Geometry check sheet. Reference: the model listing, model coordinates, mm. A direction names the side the tool comes from. Round coordinates to 2 decimals unless told otherwise and drop trailing zeros. Order: outer loops, then holes, each group sorted by start corner. A loop starts at its lowest first (then second) coordinate and runs counter-clockwise, first axis right, second up. Notation, with made-up numbers: (20.25, 43.5) -> (43.25, 43.5) arc R16 cw to (43.25, 49.5) -> close; hole circle Ø1 at (51, -22.75). An arc over 180 degrees is marked (long way). Answer as a JSON object with one key per item and string values. Group by question number.
from build123d import *

# Parameters (mm, degrees)
EXTRUDE077_DEPTH                     = 23
EXTRUDE077_PLACEMENT_ANGLE           = 45
EXTRUDE076_DEPTH                     = 23
EXTRUDE076_PLACEMENT_ANGLE           = -45
EXTRUDE049_DEPTH                     = 5
SKETCH050_AS_DRAWN_R                 = 10.75
EXTRUDE048_DEPTH                     = 27
EXTRUDE048_ONTO_SKETCH050_ROLL_ANGLE = 90
SKETCH052_R                          = 2.75
EXTRUDE050_DEPTH                     = 3
SKETCH046_R                          = 3.5
SKETCH046_R_2                        = 1.75
SKETCH046_R_3                        = 1.65
EXTRUDE044_DEPTH                     = 30
SKETCH047_AS_DRAWN_R                 = 12.5
EXTRUDE047_DEPTH                     = 50
EXTRUDE047_ONTO_SKETCH047_ROLL_ANGLE = 90
EXTRUDE045_DEPTH                     = 60
SKETCH049_AS_DRAWN_W                 = 50
SKETCH049_AS_DRAWN_H                 = 17.5
EXTRUDE046_DEPTH                     = 78
EXTRUDE046_ONTO_SKETCH049_ROLL_ANGLE = 90
CHAMFER_SIZE                         = 0.5
CHAMFER_PLACEMENT_ANGLE              = 180


with BuildPart() as extrude077:
    # Sketch077 → Extrude077 (new body)
    with BuildSketch(Plane.YZ):
        Polygon((-8.660254, 15), (0, 15), (0, 0), align=None)
    extrude(amount=-EXTRUDE077_DEPTH)


with BuildPart() as extrude077_1:
    # Extrude077 placement: moved
    add(extrude077.part.moved(Location((-13, 0, 0))).rotate(Axis((-13, 0, 0), (0, 0, 1)), EXTRUDE077_PLACEMENT_ANGLE))


with BuildPart() as fusion032:
    # Sketch077 → Extrude076 (new body)
    with BuildSketch(Plane.YZ):
        Polygon((-8.660254, 15), (0, 15), (0, 0), align=None)
    extrude(amount=EXTRUDE076_DEPTH)


with BuildPart() as fusion032_1:
    # Extrude076 placement: moved
    add(fusion032.part.moved(Location((13, 0, 0))).rotate(Axis((13, 0, 0), (0, 0, 1)), EXTRUDE076_PLACEMENT_ANGLE))

    # Fusion032: union Extrude077
    add(extrude077_1.part)


with BuildPart() as fusion032_2:
    # Fusion032 placement: moved
    add(fusion032_1.part.moved(Location((0, 59, 3))))


with BuildPart() as extrude049:
    # Sketch051 → Extrude049 (new body)
    with BuildSketch(Plane(origin=(0, 40, 0), x_dir=(1, 0, 0), z_dir=(0, 0, 1))):
        Polygon((-16, 0.25), (-13.185417, -1.375), (-13.185417, -4.625), (-16, -6.25), (-18.814583, -4.625), (-18.814583, -1.375), align=None)
        Polygon((16, 0.25), (18.814583, -1.375), (18.814583, -4.625), (16, -6.25), (13.185417, -4.625), (13.185417, -1.375), align=None)
    extrude(amount=EXTRUDE049_DEPTH)


with BuildPart() as extrude049_1:
    # Extrude049 placement: moved
    add(extrude049.part.moved(Location((0, 0, 13))))


with BuildPart() as extrude048:
    # Sketch050 as drawn → Extrude048 (new)
    with BuildSketch(Plane.XY):
        Circle(SKETCH050_AS_DRAWN_R)
    extrude(amount=-EXTRUDE048_DEPTH)


with BuildPart() as extrude048_1:
    # Extrude048 onto Sketch050 roll: moved
    add(extrude048.part.rotate(Axis((0, 0, 0), (1, 0, 0)), EXTRUDE048_ONTO_SKETCH050_ROLL_ANGLE))


with BuildPart() as extrude048_2:
    # Extrude048 onto Sketch050 placement: moved
    add(extrude048_1.part.moved(Location((0, 33, 0))))


with BuildPart() as extrude048_3:
    # Extrude048 placement: moved
    add(extrude048_2.part.moved(Location((0, -17, 0))))


with BuildPart() as extrude050:
    # Sketch052 → Extrude050 (new body)
    with BuildSketch(Plane.XY):
        with Locations((-6.717514, 6.717514)):
            Circle(SKETCH052_R)
        with Locations((5.656854, 5.656854)):
            Circle(SKETCH052_R)
        with Locations((6.717514, -6.717514)):
            Circle(SKETCH052_R)
        with Locations((-5.656854, -5.656854)):
            Circle(SKETCH052_R)
    extrude(amount=EXTRUDE050_DEPTH)


with BuildPart() as extrude050_1:
    # Extrude050 placement: moved
    add(extrude050.part.moved(Location((0, 0, 8))))


with BuildPart() as extrude044:
    # Sketch046 → Extrude044 (new body)
    with BuildSketch(Plane.XY):
        Circle(SKETCH046_R)
        with Locations((-16, 37)):
            Circle(SKETCH046_R_2)
        with Locations((16, 37)):
            Circle(SKETCH046_R_2)
        with Locations((6.717514, -6.717514)):
            Circle(SKETCH046_R_3)
        with Locations((-6.717514, 6.717514)):
            Circle(SKETCH046_R_3)
        with Locations((-5.656854, -5.656854)):
            Circle(SKETCH046_R_3)
        with Locations((5.656854, 5.656854)):
            Circle(SKETCH046_R_3)
        with BuildLine():
            ThreePointArc((4.437602, 12.5547), (0, 27.211103), (-4.437602, 12.5547))
            Line((-4.437602, 12.5547), (-1.1094, 10.335899))
            ThreePointArc((-1.1094, 10.335899), (0, 10), (1.1094, 10.335899))
            Line((4.437602, 12.5547), (1.1094, 10.335899))
        make_face()
        with BuildLine():
            Line((-20.5, 0), (-20.5, 70))
            Line((-20.5, 70), (-29.5, 70))
            Line((-29.5, 70), (-29.5, -30))
            Line((-29.5, -30), (29.5, -30))
            Line((29.5, -30), (29.5, 70))
            Line((29.5, 70), (20.5, 70))
            Line((20.5, 70), (20.5, 0))
            ThreePointArc((-20.5, 0), (0, -20.5), (20.5, 0))
        make_face()
    extrude(amount=EXTRUDE044_DEPTH)


with BuildPart() as extrude047:
    # Sketch047 as drawn → Extrude047 (new)
    with BuildSketch(Plane.XY):
        Circle(SKETCH047_AS_DRAWN_R)
    extrude(amount=-EXTRUDE047_DEPTH)


with BuildPart() as extrude047_1:
    # Extrude047 onto Sketch047 roll: moved
    add(extrude047.part.rotate(Axis((0, 0, 0), (1, 0, 0)), EXTRUDE047_ONTO_SKETCH047_ROLL_ANGLE))


with BuildPart() as extrude047_2:
    # Extrude047 onto Sketch047 placement: moved
    add(extrude047_1.part.moved(Location((0, 32, 0))))


with BuildPart() as extrude047_3:
    # Extrude047 placement: moved
    add(extrude047_2.part.moved(Location((0, -3, 0))))


with BuildPart() as extrude045:
    # Sketch048 → Extrude045 (new body)
    with BuildSketch(Plane.YZ.offset(33)):
        Polygon((-30, 8), (16, 8), (20.618802, 0), (-30, 0), align=None)
    extrude(amount=-EXTRUDE045_DEPTH)


with BuildPart() as chamfer_body:
    # Sketch049 as drawn → Extrude046 (new)
    with BuildSketch(Plane.XY):
        with Locations((0, 8.75)):
            Rectangle(SKETCH049_AS_DRAWN_W, SKETCH049_AS_DRAWN_H)
    extrude(amount=-EXTRUDE046_DEPTH)


with BuildPart() as chamfer_body_1:
    # Extrude046 onto Sketch049 roll: moved
    add(chamfer_body.part.rotate(Axis((0, 0, 0), (1, 0, 0)), EXTRUDE046_ONTO_SKETCH049_ROLL_ANGLE))


with BuildPart() as chamfer_body_2:
    # Extrude046 onto Sketch049 placement: moved
    add(chamfer_body_1.part.moved(Location((0, -28, 0))))

    # Cut029: cut Extrude045
    add(extrude045.part, mode=Mode.SUBTRACT)

    # Cut001: cut Extrude047
    add(extrude047_3.part, mode=Mode.SUBTRACT)

    # Cut030: cut Extrude044
    add(extrude044.part, mode=Mode.SUBTRACT)

    # Cut031: cut Extrude050
    add(extrude050_1.part, mode=Mode.SUBTRACT)

    # Cut004: cut Extrude048
    add(extrude048_3.part, mode=Mode.SUBTRACT)

    # Cut005: cut Extrude049
    add(extrude049_1.part, mode=Mode.SUBTRACT)

    # Cut043: cut Fusion032
    add(fusion032_2.part, mode=Mode.SUBTRACT)

    # Chamfer
    chamfer_edges = [chamfer_body_2.edges().sort_by_distance(p)[0] for p in [
        (0, -20.5, 17.5),
        (20.5, 19.8304, 17.5),
        (15.3304, 44.8304, 17.5),
        (0, 50, 17.5),
        (-15.3304, 44.8304, 17.5),
        (-20.5, 19.8304, 17.5),
        (-14.592709, 39.4375, 17.5),
        (-17.407291, 39.4375, 17.5),
        (-13.185417, 37, 17.5),
        (-18.814583, 37, 17.5),
        (-14.592709, 34.5625, 17.5),
        (-17.407291, 34.5625, 17.5),
        (-7.306854, -5.656854, 17.5),
        (-8.367514, 6.717514, 17.5),
        (0, 27.211103, 17.5),
        (-2.773501, 11.4453, 17.5),
        (2.773501, 11.4453, 17.5),
        (0, 10, 17.5),
        (-3.5, 0, 17.5),
        (14.592709, 39.4375, 17.5),
        (13.185417, 37, 17.5),
        (17.407291, 39.4375, 17.5),
        (14.592709, 34.5625, 17.5),
        (18.814583, 37, 17.5),
        (17.407291, 34.5625, 17.5),
        (4.006854, 5.656854, 17.5),
        (5.067514, -6.717514, 17.5),
        (0, -20.5, 8),
        (20.5, 18.309401, 4),
        (20.5, 8, 8),
        (20.5, 44.8304, 11.168559),
        (20.5, 50, 2.418559),
        (15.3304, 50, 11.168559),
        (0, 50, 12.5),
        (-20.5, 50, 2.418559),
        (-15.3304, 50, 11.168559),
        (-20.5, 44.8304, 11.168559),
        (-20.5, 8, 8),
        (-20.5, 18.309401, 4),
        (13.185417, 38.625, 15.25),
        (3.967514, -6.717514, 8),
        (-8.406854, -5.656854, 8),
        (2.906854, 5.656854, 8),
        (-9.467514, 6.717514, 8),
        (14.25, 37, 0),
        (-17.75, 37, 0),
    ]]
    chamfer(chamfer_edges, length=CHAMFER_SIZE)


with BuildPart() as chamfer_body_3:
    # Chamfer placement: moved
    add(chamfer_body_2.part.rotate(Axis((0, 0, 0), (0, 1, 0)), CHAMFER_PLACEMENT_ANGLE))


solid = chamfer_body_3.part
Item 1: Sectioned sample at B-B, the plane y = 37. Count the separate pieces of the cut face and the enclosed holes in it, then the cut area to 3 significant figures.
Item 2: Depth check by flat-ended pin: pin 1 Ø6 at (x, z) = (5.5, -7) entering from -Y; pin 2 Ø1.5 at (x, z) = (12, -15.5) entering from -Y; pin 3 Ø4.5 at (x, y) = (-7.5, -7) entering from +Z. Enter the tip coordinate at first touch or a pass-through.
Item 3: Mould release check, pull along Y, two halves, no side actions. Record for faces 5 (the cylindrical face through (0, 10, -12)), 6 (the flat face through (-15.16, 18.277, -4.056)), 7 (the flat face through (-20.5, 25, -8)): pulls with the +Y half, pulls with the -Y half, needs draft (parallel to the pull), parting line crosses it, or undercut.
Item 4: Thickness scan on L1, parallel to Y at x = 4.5, z = -13; L2, parallel to X at y = 0.5, z = -8.5; L3, parallel to Z at x = -11, y = 3.5. Record the ranges inside material, lowest first.
Item 5: Sectioned sample at A-A, the plane x = 0. Enter the section's corners in (y, z).
Item 6: Set-up check for faces 1 (the flat face through (0, 50, -14)), 2 (the cylindrical face through (-0.275, 39.107, -12.497)), 3 (the cylindrical face through (5.239, 9.036, -9.732)), 4 (the flat face through (-13.185, 37, -15)): record each of +Z, -Z, +X, -X, +Y, -Y from which the full face is reachable in a straight line by a thin tool's end or side.
Result:
{
 "1": {"separate pieces": "3", "enclosed holes": "0", "area": "329 mm2"},
 "2": {"pin 1": "stops at y = -20.29", "pin 2": "stops at y = -17.14", "pin 3": "stops at z = -8.17"},
 "3": {"face 5": "undercut", "face 6": "pulls with the -Y half", "face 7": "needs draft"},
 "4": {"L1": "y = -20 to -6.83, -4.48 to 12.6, 25.83 to 50", "L2": "x = -20.5 to -3.46, 3.46 to 20.5", "L3": "z = -17.5 to -8"},
 "5": {"outline": "(-20.5, -17) -> (-20, -17.5) -> (-4, -17.5) -> (-3.5, -17) -> (-3.5, -8) -> (-20, -8) -> (-20.5, -8.5) -> close; (3.5, -17) -> (4, -17.5) -> (9.5, -17.5) -> (10, -17) -> (10, -8) -> (3.5, -8) -> close; (27.21, -17) -> (27.71, -17.5) -> (49.5, -17.5) -> (50, -17) -> (50, -13) -> (49.5, -12.5) -> (29, -12.5) -> (29, -10.75) -> (27.21, -10.75) -> close"},
 "6": {"face 1": "+Z, -Z, +X, -X, +Y", "face 2": "+Z, +Y", "face 3": "+Z", "face 4": "-Z"}
}
